Part model, mm, in its own coordinate system. Face numbers are marked on the shaded views. A direction names the side the tool comes from. Round coordinates to 2 decimals unless told otherwise and drop trailing zeros. Write each loop counter-clockwise with the first axis right and the second up, starting at its lowest first coordinate (ties: lowest second). Pieces come first, ordered by that corner, then holes.
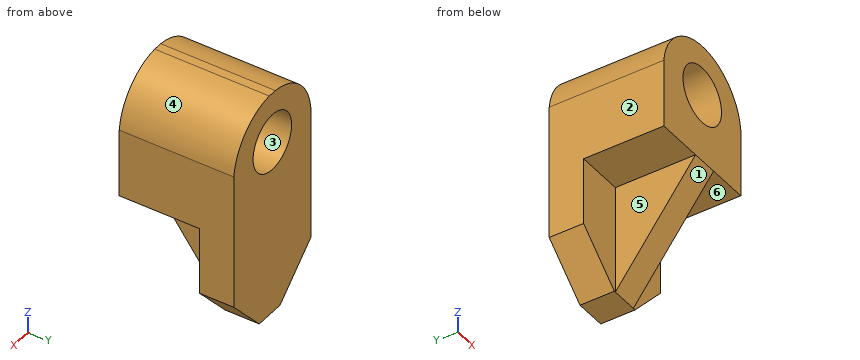
from build123d import *

# Parameters (mm, degrees)
F0_W     = 762
F0_H     = 1524
F1_DEPTH = 762
F4_DEPTH = 762.001
F5_DEPTH = 762.001
F6_DEPTH = 533.4
F8_DEPTH = 447.422


with BuildPart() as f1:
    # F0 (on Front) → F1 (new body)
    with BuildSketch(Plane.XZ):
        with Locations((381, -762)):
            Rectangle(F0_W, F0_H)
    extrude(amount=F1_DEPTH)

    # F3 (on face) + F2 (on face) → F4 (cut, through all)
    with BuildSketch(Plane.XZ.offset(762)):
        Polygon((762, -1246.666074), (509.469922, -1524), (762, -1524), align=None)
        Polygon((304.574043, -1524), (0, -1246.666074), (0, -1524), align=None)
    with BuildSketch(Plane.XZ.offset(762)):
        with BuildLine():
            Line((762, 0), (410.814423, 0))
            ThreePointArc((410.814423, 0), (647.486394, -106.600051), (762, -339.546025))
            Line((762, -339.546025), (762, 0))
        make_face()
        with BuildLine():
            Line((0, 0), (0, -339.546025))
            ThreePointArc((0, -339.546025), (114.513606, -106.600051), (351.185577, 0))
            Line((351.185577, 0), (0, 0))
        make_face()
    extrude(amount=-F4_DEPTH, mode=Mode.SUBTRACT)

    # F2 (on face) → F5 (cut, through all)
    with BuildSketch(Plane.XZ.offset(762)):
        with BuildLine():
            Line((380.433679, -339.546025), (189.933679, -339.546025))
            ThreePointArc((189.933679, -339.546025), (380.433679, -530.046025), (570.933679, -339.546025))
            Line((570.933679, -339.546025), (380.433679, -339.546025))
        make_face()
        with BuildLine():
            ThreePointArc((570.933679, -339.546025), (380.433679, -149.046025), (189.933679, -339.546025))
            Line((189.933679, -339.546025), (380.433679, -339.546025))
            Line((380.433679, -339.546025), (570.933679, -339.546025))
        make_face()
    extrude(amount=-F5_DEPTH, mode=Mode.SUBTRACT)

    # F2 (on face) → F6 (cut)
    with BuildSketch(Plane.XZ.offset(762)):
        Polygon((492.379, -796.746025), (492.379, -1524), (533.4, -1524), (762, -1524), (762, -1382.540822), (762, -796.746025), align=None)
        Polygon((0, -796.746025), (0, -1524), (228.6, -1524), (314.579, -1524), (314.579, -796.746025), align=None)
    extrude(amount=-F6_DEPTH, mode=Mode.SUBTRACT)

    # F7 (on face) → F8 (cut, through all)
    with BuildSketch(Plane(origin=(314.579, 0, 0), x_dir=(0, -1, 0), z_dir=(-1, 0, 0))):
        Polygon((762, -1524), (762, -796.746025), (228.6, -1524), align=None)
    extrude(amount=-F8_DEPTH, mode=Mode.SUBTRACT)


solid = f1.part
Q1. Tool access for the marked faces 4, 5 and 6: list every direction of +Z, -Z, +X, -X, +Y, -Y with a clear straight run to the whole face (end or side of a thin tool).
Q2. Drop flat-ended pins along their axis: P1, Ø3, axis at x = 299.5, y = -547.5, coming from the -Z side; P2, Ø12, axis at x = 359, y = -459, coming from the -Z side; P3, Ø2, axis at y = -371.5, z = -1294.5, coming from the -X side. Give the stop position or say it passes through.
Q3. Saw through at D-D, the plane x = 541. Write the cut outline in (y, z), and give its area (3 significant figures).
Q4. Saw through at C-C, the plane z = -436. Write the cut outline in (x, y), and give its area (3 significant figures).
Q5. Two-plate mould, pull along X, no slides. Class the marked faces 1, 2 and 3: released by +X, released by -X, zero draft, split by the parting line, or undercut.
Q6. Wall check: line 1 (Y direction, x = 146.5, z = -1173); line 2 (Z direction, x = 286, y = -396); line 3 (X direction, y = -115, z = -368.5). Give the ranges that are in metal, low to high.
Q7. Saw through at A-A, the plane x = 242. Write the cut outline in (y, z), and give its area (3 significant figures).
Q8. Saw through at B-B, the plane y = -166.5. Write the cut outline in (x, z), and give its area (3 significant figures).
Computed:
1. face 4: +Z, +X, +Y, -Y
1. face 5: -Z, -X, -Y
1. face 6: -Z, +X, -Y
2. P1: stops at z = -796.75
2. P2: stops at z = -1218.05
2. P3: stops at x = 314.58
3. outline: (-762, -796.75) - (-228.6, -796.75) - (-228.6, -1489.37) - (0, -1489.37) - (0, -442.06) - (-762, -442.06) - close; (-762, -237.03) - (0, -237.03) - (0, -33.82) - (-762, -33.82) - close
3. area: 583,000 mm2
4. outline: (0, -762) - (216.16, -762) - (216.16, 0) - (0, 0) - close; (544.71, -762) - (762, -762) - (762, 0) - (544.71, 0) - close
4. area: 330,000 mm2
5. face 1: zero draft
5. face 2: released by -X
5. face 3: undercut
6. line 1: y = -228.6 to 0
6. line 2: z = -796.75 to -504.99, -174.1 to -10.8
6. line 3: x = 0 to 192.15, 568.72 to 762
7. outline: (-762, -796.75) - (-228.6, -796.75) - (-228.6, -1467.02) - (0, -1467.02) - (0, -470.41) - (-762, -470.41) - close; (-762, -208.68) - (0, -208.68) - (0, -24.92) - (-762, -24.92) - close
7. area: 542,000 mm2
8. outline: (0, -1246.67) - (304.57, -1524) - (509.47, -1524) - (762, -1246.67) - (762, -339.55) arc R383.38 ccw to (410.81, 0) - (351.19, 0) arc R383.38 ccw to (0, -339.55) - close; hole circle Ø381 at (380.43, -339.55)
8. area: 909,000 mm2
